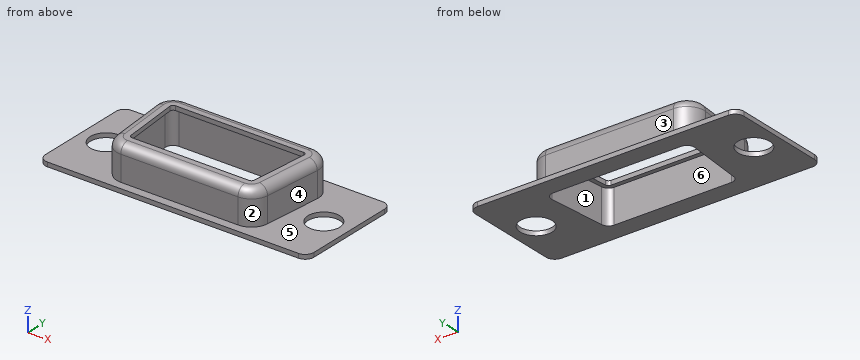
from build123d import *

# Parameters (mm, degrees)
BOSS_EXTRUDE1_DEPTH = 0.5
SKETCH2_R           = 1.825
CUT_EXTRUDE1_DEPTH  = 0.5
BOSS_EXTRUDE2_DEPTH = 3.9
CUT_EXTRUDE2_DEPTH  = 4.4
CUT_EXTRUDE3_DEPTH  = 3.9
FILLET1_R           = 1


with BuildPart() as part:
    # Sketch1 → Boss-Extrude1 (new body)
    with BuildSketch(Plane.XY):
        with BuildLine():
            Line((-14.42, 6.275), (14.42, 6.275))
            ThreePointArc((14.42, 6.275), (15.127106781, 5.982106781), (15.42, 5.275))
            Line((15.42, 5.275), (15.42, -5.275))
            ThreePointArc((15.42, -5.275), (15.127106781, -5.982106781), (14.42, -6.275))
            Line((14.42, -6.275), (-14.42, -6.275))
            ThreePointArc((-14.42, -6.275), (-15.127106781, -5.982106781), (-15.42, -5.275))
            Line((-15.42, -5.275), (-15.42, 5.275))
            ThreePointArc((-15.42, 5.275), (-15.127106781, 5.982106781), (-14.42, 6.275))
        make_face()
    extrude(amount=BOSS_EXTRUDE1_DEPTH)

    # Sketch2 → Cut-Extrude1 (cut)
    with BuildSketch(Plane.XY.offset(0.5)):
        with Locations((-12.495, 0)):
            Circle(SKETCH2_R)
        with Locations((12.495, 0)):
            Circle(SKETCH2_R)
    extrude(amount=-CUT_EXTRUDE1_DEPTH, mode=Mode.SUBTRACT)

    # Sketch3 → Boss-Extrude2 (add)
    with BuildSketch(Plane.XY.offset(0.5)):
        with BuildLine():
            Line((-7.352440505, 5.3), (7.352440505, 5.3))
            ThreePointArc((7.352440505, 5.3), (8.831577141, 4.646162996), (9.34359951, 3.112154811))
            Line((9.34359951, 3.112154811), (8.720958001, -3.487845189))
            ThreePointArc((8.720958001, -3.487845189), (8.075961991, -4.779136636), (6.729798996, -5.3))
            Line((6.729798996, -5.3), (-6.729798996, -5.3))
            ThreePointArc((-6.729798996, -5.3), (-8.075961991, -4.779136636), (-8.720958001, -3.487845189))
            Line((-8.720958001, -3.487845189), (-9.34359951, 3.112154811))
            ThreePointArc((-9.34359951, 3.112154811), (-8.831577141, 4.646162996), (-7.352440505, 5.3))
        make_face()
    extrude(amount=BOSS_EXTRUDE2_DEPTH)

    # Sketch4 → Cut-Extrude2 (cut)
    with BuildSketch(Plane.XY.offset(4.4)):
        with BuildLine():
            Line((7.078251822, -3.332872908), (7.700893331, 3.267127092))
            ThreePointArc((7.700893331, 3.267127092), (7.611289416, 3.535578524), (7.352440505, 3.65))
            Line((7.352440505, 3.65), (-7.352440505, 3.65))
            ThreePointArc((-7.352440505, 3.65), (-7.611289416, 3.535578524), (-7.700893331, 3.267127092))
            Line((-7.700893331, 3.267127092), (-7.078251822, -3.332872908))
            ThreePointArc((-7.078251822, -3.332872908), (-6.96537752, -3.558848911), (-6.729798996, -3.65))
            Line((-6.729798996, -3.65), (6.729798996, -3.65))
            ThreePointArc((6.729798996, -3.65), (6.96537752, -3.558848911), (7.078251822, -3.332872908))
        make_face()
    extrude(amount=-CUT_EXTRUDE2_DEPTH, mode=Mode.SUBTRACT)

    # Sketch5 → Cut-Extrude3 (cut)
    with BuildSketch(Plane.XY.offset(3.9)):
        with BuildLine():
            Line((7.352440505, 4.15), (-7.352440505, 4.15))
            ThreePointArc((-7.352440505, 4.15), (-7.981073576, 3.872119273), (-8.198683082, 3.220165795))
            Line((-8.198683082, 3.220165795), (-7.576041573, -3.379834205))
            ThreePointArc((-7.576041573, -3.379834205), (-7.301918269, -3.92863307), (-6.729798996, -4.15))
            Line((-6.729798996, -4.15), (6.729798996, -4.15))
            ThreePointArc((6.729798996, -4.15), (7.301918269, -3.92863307), (7.576041573, -3.379834205))
            Line((7.576041573, -3.379834205), (8.198683082, 3.220165795))
            ThreePointArc((8.198683082, 3.220165795), (7.981073576, 3.872119273), (7.352440505, 4.15))
        make_face()
        with BuildLine():
            Line((7.352440505, 3.65), (-7.352440505, 3.65))
            ThreePointArc((-7.352440505, 3.65), (-7.611289416, 3.535578524), (-7.700893331, 3.267127092))
            Line((-7.700893331, 3.267127092), (-7.078251822, -3.332872908))
            ThreePointArc((-7.078251822, -3.332872908), (-6.96537752, -3.558848911), (-6.729798996, -3.65))
            Line((-6.729798996, -3.65), (6.729798996, -3.65))
            ThreePointArc((6.729798996, -3.65), (6.96537752, -3.558848911), (7.078251822, -3.332872908))
            Line((7.078251822, -3.332872908), (7.700893331, 3.267127092))
            ThreePointArc((7.700893331, 3.267127092), (7.611289416, 3.535578524), (7.352440505, 3.65))
        make_face(mode=Mode.SUBTRACT)
    extrude(amount=-CUT_EXTRUDE3_DEPTH, mode=Mode.SUBTRACT)

    # Fillet1
    fillet1_edges = [part.edges().sort_by_distance(p)[0] for p in [
        (8.075961991, -4.779136636, 4.4),
        (9.032278756, -0.187845189, 4.4),
        (8.831577141, 4.646162996, 4.4),
        (0, 5.3, 4.4),
        (-8.831577141, 4.646162996, 4.4),
        (-9.032278756, -0.187845189, 4.4),
        (-8.075961991, -4.779136636, 4.4),
        (0, -5.3, 4.4),
    ]]
    fillet(fillet1_edges, radius=FILLET1_R)


solid = part.part
Model file for the job. Use its own axes, mm. Face numbers are marked on the shaded views. A direction names the side the tool comes from. Give positions to 0.01 mm unless a question says otherwise; leave off trailing zeros. Order: outer loops, then holes, each group sorted by start corner. A loop starts at its lowest first (then second) coordinate and runs counter-clockwise, first axis right, second up. Notation, with made-up numbers: (83, 72.25) - (119, 72.25) arc R26 cw to (119, 88.25) - close; hole circle Ø8 at (-4, -37). An arc over 180 degrees is marked (long way). Write item = value, one per line. Start each with the question number.
1. Cut at A-A, the plane z = 3.1. List the corners of the cut face in (x, y).
2. Drop flat-ended pins along their axis: P1, Ø2, axis at x = 1, z = 2.5, coming from the -Y side; P2, Ø1.5, axis at x = 0, z = 2, coming from the +Y side. Give the stop position or say it passes through.
3. Which spindle directions (+Z, -Z, +X, -X, +Y, -Y) get a long thin tool onto all of the face, cutting with end or side? Do the marked faces 1, 2 and 3. Say none if no direction does.
4. Cut at C-C, the plane y = 0. State how many separate pieces and enclosed holes the cut face has, and give its area (3 significant figures).
5. Probe line 1 along Y through (x, z) = (1.5, 0.9); line 2 along X through (y, z) = (-0.5, 0.2); line 3 along X through (y, z) = (-2, 1.8). List the from-to ranges inside material, lowest first.
6. Cut at B-B, the plane x = -10. List the corners of the cut face in (y, z) (3 decimals).
7. Two-plate mould, pull along X, no slides. Class the marked faces 4, 5 and 6: pulls with the +X half, pulls with the -X half, needs draft (parallel to the pull), parting line crosses it, or undercut.
Taken from the geometry:
q1.outline = (-9.34, 3.11) - (-8.72, -3.49) arc R2 ccw to (-6.73, -5.3) - (6.73, -5.3) arc R2 ccw to (8.72, -3.49) - (9.34, 3.11) arc R2 ccw to (7.35, 5.3) - (-7.35, 5.3) arc R2 ccw to start; hole (-8.2, 3.22) - (-7.58, -3.38) arc R0.85 ccw to (-6.73, -4.15) - (6.73, -4.15) arc R0.85 ccw to (7.58, -3.38) - (8.2, 3.22) arc R0.85 ccw to (7.35, 4.15) - (-7.35, 4.15) arc R0.85 ccw to start
q2.P1 = -5.3
q2.P2 = 5.3
q3.face_1 = -Z
q3.face_2 = +Z, +X, -Y
q3.face_3 = +Z, +X, -X, +Y
q4.separate_pieces = 4
q4.enclosed_holes = 0
q4.area = 13.0 mm²
q5.line_1 = -5.3 to -4.15, 4.15 to 5.3
q5.line_2 = -15.42 to -14.25, -10.74 to -7.85, 7.85 to 10.74, 14.25 to 15.42
q5.line_3 = -8.86 to -7.71, 7.71 to 8.86
q6.outline = (-6.275, 0) - (6.275, 0) - (6.275, 0.5) - (-6.275, 0.5) - close
q7.face_4 = pulls with the +X half
q7.face_5 = needs draft
q7.face_6 = undercut
